CAD build for the part. Positions are in the model's coordinates, mm. Face numbers are marked on the shaded views. A direction names the side the tool comes from. Round coordinates to 2 decimals unless told otherwise and drop trailing zeros. Write each loop counter-clockwise with the first axis right and the second up, starting at its lowest first coordinate (ties: lowest second). Pieces come first, ordered by that corner, then holes. Notation, with made-up numbers: (-39.5, 54.5) - (12.5, 54.5) arc R20 cw to (12.5, 93.5) - close; hole circle Ø8 at (61, 23.25). An arc over 180 degrees is marked (long way). Answer in a Markdown table with one row per item.
```python
from build123d import *

# Parameters (mm, degrees)
F0_W     = 50.8
F0_H     = 50.8
F1_DEPTH = 50.8
F2_R     = 12.7
F3_DEPTH = 12.7
F4_W     = 20.050239
F4_H     = 18.331647
F5_DEPTH = 12.7
F6_R     = 12.7
F7_DEPTH = 50.8


with BuildPart() as f1:
    # F0 (on Front) → F1 (new body)
    with BuildSketch(Plane.XZ):
        with Locations((25.4, 25.4)):
            Rectangle(F0_W, F0_H)
    extrude(amount=F1_DEPTH)

    # F2 (on face) → F3 (join)
    with BuildSketch(Plane.XZ.offset(50.8)):
        with Locations((25.206016, 25.778878)):
            Circle(F2_R)
    extrude(amount=F3_DEPTH)

    # F4 (on face) → F5 (join)
    with BuildSketch(Plane.YZ.offset(50.8)):
        with Locations((-26.06531, 26.160787)):
            Rectangle(F4_W, F4_H)
    extrude(amount=F5_DEPTH)

    # F6 (on face) → F7 (cut)
    with BuildSketch(Plane.XY.offset(50.8)):
        with Locations((26.733654, -25.587924)):
            Circle(F6_R)
    extrude(amount=-F7_DEPTH, mode=Mode.SUBTRACT)


solid = f1.part
```
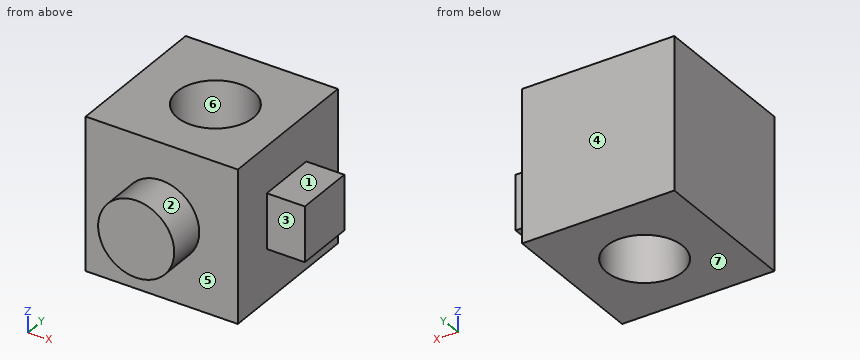
Q1. Drill centre lines: line 1 (Y direction, x = 6, z = 47.5); line 2 (X direction, y = -47.5, z = 4); line 3 (X direction, y = -37, z = 15.5). Where is each one in solid material? Low to high.
Computed:
| item | result |
|---|---|
| line 1 | y = -50.8 to 0 |
| line 2 | x = 0 to 50.8 |
| line 3 | x = 0 to 21.16, 32.31 to 50.8 |
Q2. Saw through at C-C on z = 34.5. List the corners of the cut face in (x, y).
Computed:
| item | result |
|---|---|
| outline | (0, -50.8) - (15.97, -50.8) - (15.97, -63.5) - (34.44, -63.5) - (34.44, -50.8) - (50.8, -50.8) - (50.8, -36.09) - (63.5, -36.09) - (63.5, -16.04) - (50.8, -16.04) - (50.8, 0) - (0, 0) - close; hole circle Ø25.4 at (26.73, -25.59) |
Q3. Flat gauge pins, fed straight in: pin 1 (14 mm diameter, centred on x = 57, z = 26, fed in from -Y); pin 2 (6.5 mm diameter, centred on x = 56, y = -28.5, fed in from -Z); pin 3 (12 mm diameter, centred on y = -56, z = 38.5, fed in from +X). Where does each tip first touch, or does it go through?
Computed:
| item | result |
|---|---|
| pin 1 | stops at y = -50.8 |
| pin 2 | stops at z = 16.99 |
| pin 3 | stops at x = 50.8 |
Q4. 3-axis set-ups, long thin cutter, end or side, ignore diameter. For the marked faces 1, 2 and 3: which of +Z, -Z, +X, -X, +Y, -Y reach the whole face in a straight line?
Computed:
| item | result |
|---|---|
| face 1 | +Z, +X, +Y, -Y |
| face 2 | -Y |
| face 3 | +Z, -Z, +X, -Y |
Q5. Saw through at B-B on x = 20. List the corners of the cut face in (y, z), then the cut area to 3 significant figures.
Computed:
| item | result |
|---|---|
| outline | (-63.5, 14.19) - (-50.8, 14.19) - (-50.8, 0) - (-36.36, 0) - (-36.36, 50.8) - (-50.8, 50.8) - (-50.8, 37.36) - (-63.5, 37.36) - close; (-14.82, 0) - (0, 0) - (0, 50.8) - (-14.82, 50.8) - close |
| area | 1,780 mm2 |
Q6. Saw through at D-D on x = 42. List the corners of the cut face in (y, z), then the cut area to 3 significant figures.
Computed:
| item | result |
|---|---|
| outline | (-50.8, 0) - (0, 0) - (0, 50.8) - (-50.8, 50.8) - close |
| area | 2,580 mm2 |
Q7. Saw through at A-A on y = -21.5. List the corners of the cut face in (x, z), then the cut area to 3 significant figures.
Computed:
| item | result |
|---|---|
| outline | (0, 0) - (14.71, 0) - (14.71, 50.8) - (0, 50.8) - close; (38.76, 0) - (50.8, 0) - (50.8, 16.99) - (63.5, 16.99) - (63.5, 35.33) - (50.8, 35.33) - (50.8, 50.8) - (38.76, 50.8) - close |
| area | 1,590 mm2 |
Q8. Pull direction Y, two halves, no side cores. Call the marked faces 4, 5, 6 and 7: released by +Y, released by -Y, zero draft, split by the parting line, or undercut.
Computed:
| item | result |
|---|---|
| face 4 | released by +Y |
| face 5 | released by -Y |
| face 6 | undercut |
| face 7 | zero draft |
